from build123d import *

# Parameters (mm, degrees)
BASE_FLANGE1_DEPTH      = 457.2
CUT_EXTRUDE1_DEPTH      = 648.7
CUT_EXTRUDE1_DEPTH_BACK = 648.7


# Sheet-metal steps are written as plain solids
with BuildPart() as part:
    # Sketch1 → Base-Flange1 (new body)
    with BuildSketch(Plane(origin=(0, 0, 0), x_dir=(0, 0, -1), z_dir=(1, 0, 0))):
        with BuildLine():
            Line((-304.8, 0), (-0.129882454, 0))
            ThreePointArc((-0.129882454, 0), (-0.001973206, 0.011190609), (0.122049584, 0.044422416))
            Line((0.122049584, 0.044422416), (104.030764306, 37.864101655))
            ThreePointArc((104.030764306, 37.864101655), (104.689368087, 38.040574007), (105.368610299, 38.1))
            Line((105.368610299, 38.1), (457.2, 38.1))
            Line((457.2, 38.1), (457.2, 34.925))
            Line((457.2, 34.925), (105.368610299, 34.925))
            ThreePointArc((105.368610299, 34.925), (105.240701051, 34.913809391), (105.116678261, 34.880577584))
            Line((105.116678261, 34.880577584), (1.207963539, -2.939101655))
            ThreePointArc((1.207963539, -2.939101655), (0.549359758, -3.115574007), (-0.129882454, -3.175))
            Line((-0.129882454, -3.175), (-304.8, -3.175))
            Line((-304.8, -3.175), (-304.8, 0))
        make_face()
    extrude(amount=BASE_FLANGE1_DEPTH)

    # Sketch6 → Cut-Extrude1 (cut, two sides: drawn at the far end of the back side and taken through both)
    with BuildSketch(Plane(origin=(0, 0, 0), x_dir=(1, 0, 0), z_dir=(0, 1, 0)).offset(-CUT_EXTRUDE1_DEPTH_BACK)):
        Polygon((0, -304.8), (76.2, -304.8), (0, -20.417728463), align=None)
        Polygon((0, 335.182271537), (0, 457.2), (85.437733265, 457.2), align=None)
        Polygon((457.2, 457.2), (371.762266735, 457.2), (457.2, 335.182271537), align=None)
        Polygon((381, -304.8), (457.2, -20.417728463), (457.2, -304.8), align=None)
    extrude(amount=CUT_EXTRUDE1_DEPTH + CUT_EXTRUDE1_DEPTH_BACK, mode=Mode.SUBTRACT)


solid = part.part
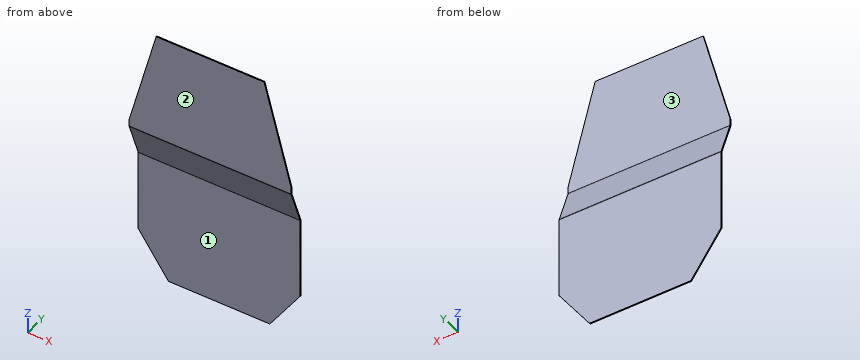
For this review, take the finished solid that the model builds, in its own axes (mm). Face numbers are marked on the shaded views. A direction names the side the tool comes from. Give positions to 0.01 mm unless a question says otherwise; leave off trailing zeros. Loops run counter-clockwise (first coordinate to the right, second up) from the corner with the lowest first, then second, coordinate; pieces in that order, holes last.
Item 1: Insertion check: pin 1 (4 mm diameter, centred on x = 385, z = -357, fed in from -Y) (3 decimals); pin 2 (8 mm diameter, centred on x = 125, z = 73, fed in from +Y). Each pin has a flat end and moves straight along its axis. Give the tip position at first contact, or say it passes through.
Item 2: Tool access review of the marked faces 1, 2 and 3: name each direction out of +Z, -Z, +X, -X, +Y, -Y from which nothing blocks a thin tool from reaching the whole face with its end or side.
Item 3: Take a section at A-A, the plane x = 163. State the section outline as (y, z) points (3 decimals).
Item 4: Take a section at B-B, the plane z = -233. State the section outline as (x, y) points (3 decimals), and give its area (3 significant figures).
Item 5: For line 1 along Y through (x, z) = (262.5, -378) (3 decimals); line 2 along Y through (x, z) = (220.5, 165) (3 decimals); line 3 along X through (y, z) = (-0.5, 216), list the stretches that pass through material, from the lowest coordinate up.
Item 6: Take a section at C-C, the plane y = 13. State the section outline as (x, z) points.
Item 7: Take a section at D-D, the plane x = 394.5. State the section outline as (y, z) points (3 decimals).
Calculated:
1. pin 1: stops at y = 34.925
1. pin 2: stops at y = 0
2. face 1: -Z, +X, -X, -Y
2. face 2: +Z, -Z, +X, -X, -Y
2. face 3: +Z, +X, -X, +Y
3. outline: (-3.175, 0.13) arc R3.912 ccw to (-2.939, -1.208) - (34.881, -105.117) arc R0.737 cw to (34.925, -105.369) - (34.925, -457.2) - (38.1, -457.2) - (38.1, -105.369) arc R3.912 ccw to (37.864, -104.031) - (0.044, -0.122) arc R0.737 cw to (0, 0.13) - (0, 304.8) - (-3.175, 304.8) - close
4. outline: (0, 34.925) - (457.2, 34.925) - (457.2, 38.1) - (0, 38.1) - close
4. area: 1,450 mm2
5. line 1: y = 34.925 to 38.1
5. line 2: y = -3.175 to 0
5. line 3: x = 52.41 to 404.79
6. outline: (0, -45) - (457.2, -45) - (457.2, -35.72) - (0, -35.72) - close
7. outline: (-3.175, 0.13) arc R3.912 ccw to (-2.939, -1.208) - (34.881, -105.117) arc R0.737 cw to (34.925, -105.369) - (34.925, -424.727) - (38.1, -424.727) - (38.1, -105.369) arc R3.912 ccw to (37.864, -104.031) - (0.044, -0.122) arc R0.737 cw to (0, 0.13) - (0, 254.417) - (-3.175, 254.417) - close
